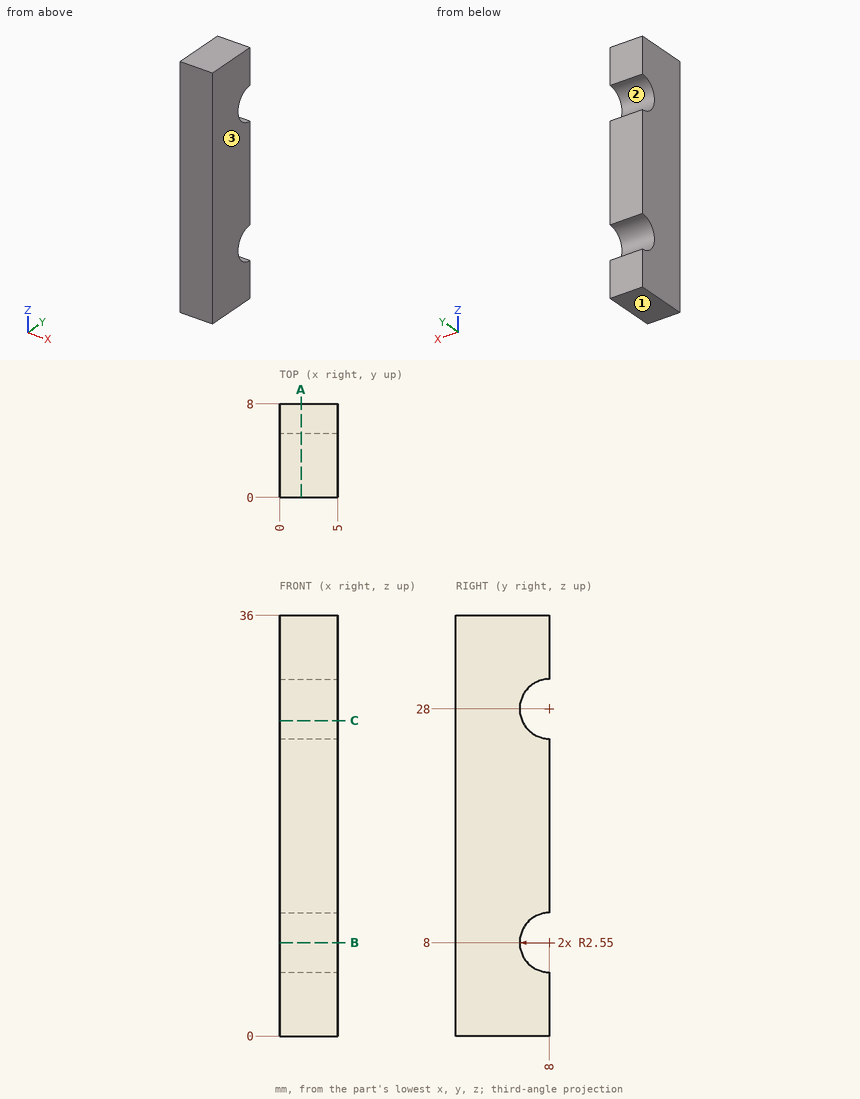
Could you check a few things on this drawing? It's one solid part, dimensions in mm from its lowest x, y, z. Give positions to 0.01 mm unless a question says otherwise; leave off trailing zeros. Write each loop counter-clockwise with the first axis right and the second up, starting at its lowest first coordinate (ties: lowest second). Pieces come first, ordered by that corner, then holes. Notation, with made-up numbers: M 43.5,-30 L 79.5,-30 A27 cw 79.5,9 Z; hole C -10,63 d8. An arc over 180 degrees is marked long. Put each result on its own line as item: value. Start each with the question number.
Item 1: I need wall thicknesses on L1, parallel to Z at x = 0.7, y = 6.75; L2, parallel to Z at x = 4, y = 5.75; L3, parallel to Y at x = 1.65, z = 8. Which ranges of each line are inside material? Lowest first, please. Write a range as from..to.
Item 2: If we section it at B-B, the plane z = 8: Write out the boundary of the cut face in (x, y), then the cut area to 4 significant figures.
Item 3: Thinking about a two-plate mould opening in Z: for the marked faces 1, 2 and 3, which applies, +Z half, -Z half, draft (parallel to the pull), parting line (faces both ways), or undercut?
Item 4: If we section it at A-A, the plane x = 1.85: Write out the boundary of the cut face in (y, z).
Item 5: If we section it at C-C, the plane z = 27: Write out the boundary of the cut face in (x, y).
Values:
1. L1: 0..5.78, 10.22..25.78, 30.22..36
1. L2: 0..6.8, 9.2..26.8, 29.2..36
1. L3: 0..5.45
2. outline: M 0,0 L 5,0 L 5,5.45 L 0,5.45 Z
2. area: 27.25 mm²
3. face 1: -Z half
3. face 2: undercut
3. face 3: draft
4. outline: M 0,0 L 8,0 L 8,5.45 A2.55 cw 8,10.55 L 8,25.45 A2.55 cw 8,30.55 L 8,36 L 0,36 Z
5. outline: M 0,0 L 5,0 L 5,5.65 L 0,5.65 Z
